from build123d import *

# Parameters (mm, degrees)
SKETCH_1_W               = 114
SKETCH_1_H               = 110
EXTRUDE_2_DEPTH          = 2.5
SKETCH_2_R               = 5
CUT_EXTRUDE_1_DEPTH      = 80.366239674
MIRROR_2_COPY_1_SKETCH_R = 5
MIRROR_2_COPY_1_DEPTH    = 80.366239674
HOLE_WIZARD_M4_1_D       = 3.3
HOLE_WIZARD_M8_3_D       = 6.8
SKETCH_8_R               = 4
CUT_EXTRUDE_2_DEPTH      = 80.366239674
HOLE_WIZARD_M8_4_D       = 6.8


with BuildPart() as part:
    # 草图1 → 凸台-拉伸2 (new, symmetric)
    with BuildSketch(Plane.XY):
        Rectangle(SKETCH_1_W, SKETCH_1_H)
    extrude(amount=EXTRUDE_2_DEPTH, both=True)

    # 草图2 → 切除-拉伸1 (cut, through all)
    with BuildSketch(Plane.XY.offset(2.5)):
        with Locations((-48, 47.5)):
            Circle(SKETCH_2_R)
    cut_extrude_1 = extrude(amount=-CUT_EXTRUDE_1_DEPTH, mode=Mode.SUBTRACT)

    # 镜向1: 切除-拉伸1 across plane
    add(cut_extrude_1.mirror(Plane.ZX), mode=Mode.SUBTRACT)

    # 镜向2: 切除-拉伸1 across plane
    add(cut_extrude_1.mirror(Plane(origin=(0, 0, 0), x_dir=(0, 0, 1), z_dir=(1, 0, 0))), mode=Mode.SUBTRACT)

    # 镜向2 copy 1 sketch → 镜向2 copy 1 (cut, through all)
    with BuildSketch(Plane(origin=(0, 0, 2.5), x_dir=(-1, 0, 0), z_dir=(0, 0, 1))):
        with Locations((-48, 47.5)):
            Circle(MIRROR_2_COPY_1_SKETCH_R)
    extrude(amount=-MIRROR_2_COPY_1_DEPTH, mode=Mode.SUBTRACT)

    # M4 螺纹孔的螺纹孔钻头1 (through all)
    with Locations(Plane(origin=(-23, 9, 2.5), x_dir=(1, 0, 0), z_dir=(0, 0, 1))):
        with Locations((0, 0), (0, -15)):
            hole_wizard_m4_1 = Hole(HOLE_WIZARD_M4_1_D / 2)

    # 镜向4: M4 螺纹孔的螺纹孔钻头1 across plane
    add(hole_wizard_m4_1.mirror(Plane(origin=(0, 0, 0), x_dir=(0, 0, 1), z_dir=(1, 0, 0))), mode=Mode.SUBTRACT)

    # M8 螺纹孔的螺纹孔钻头3 (through all)
    with Locations(Plane(origin=(0, 33, 2.5), x_dir=(1, 0, 0), z_dir=(0, 0, 1))):
        with Locations((0, 0)):
            Hole(HOLE_WIZARD_M8_3_D / 2)

    # 草图8 → 切除-拉伸2 (cut, through all)
    with BuildSketch(Plane.XY.offset(2.5)):
        with Locations((0, 47.5)):
            Circle(SKETCH_8_R)
    extrude(amount=-CUT_EXTRUDE_2_DEPTH, mode=Mode.SUBTRACT)

    # M8 螺纹孔的螺纹孔钻头4 (through all)
    with Locations(Plane(origin=(0, -47.5, 2.5), x_dir=(1, 0, 0), z_dir=(0, 0, 1))):
        with Locations((0, 0)):
            Hole(HOLE_WIZARD_M8_4_D / 2)


solid = part.part
For this review, take the finished solid that the model builds, in its own axes (mm). Coordinates: 2 decimals unless noted, no trailing zeros. Loops run counter-clockwise (first coordinate to the right, second up) from the corner with the lowest first, then second, coordinate; pieces in that order, holes last. Notation, with made-up numbers: (13.25, 23.5) - (18.25, 23.5) arc R13 ccw to (18.25, 43.5) - close; hole circle Ø11 at (40.5, 63). An arc over 180 degrees is marked (long way). Use a Markdown table: item, result. Add a question column.
Item 1: We need section D-D (z = 0.65). Give the number of separate pieces and of enclosed holes in the cut face, and give its area (3 significant figures).
Item 2: Insertion check: pin 1 Ø6 at (x, y) = (0, -47.5) entering from -Z. The pin has a flat end and moves straight along its axis. Give the tip position at first contact, or say it passes through.
Item 3: We need section A-A (x = 0). Give the boundary of the cut face in (y, z), and give its area (3 significant figures).
Item 4: Mouldability with a two-part tool opening along Y and no side actions: class faces 1 (the face through (-1, -55, 0)), 2 (the face through (-57, -1, 0)), 3 (the face through (-21.69, 8, -0.03)), 4 (the face through (-1, 55, 0)) as pulls with the +Y half, pulls with the -Y half, needs draft (parallel to the pull), parting line crosses it, or undercut.
Item 5: We need section B-B (y = -47.5). Give the boundary of the cut face in (x, z), and give its area (3 significant figures).
Item 6: We need section C-C (x = 23). Give the boundary of the cut face in (y, z).
Item 7: For line 1 (Y direction, x = -23, z = 1.4); line 2 (X direction, y = -45.5, z = 2); line 3 (Y direction, x = 1.5, z = 0.2), list the stretches that pass through material, from the lowest coordinate up.
Results list:
| question | item | result |
|---|---|---|
| 1 | separate pieces | 1 |
| 1 | enclosed holes | 11 |
| 1 | area | 12,100 mm^2 |
| 2 | pin 1 | passes through |
| 3 | outline | (-55, -2.5) - (-50.9, -2.5) - (-50.9, 2.5) - (-55, 2.5) - close; (-44.1, -2.5) - (29.6, -2.5) - (29.6, 2.5) - (-44.1, 2.5) - close; (36.4, -2.5) - (43.5, -2.5) - (43.5, 2.5) - (36.4, 2.5) - close; (51.5, -2.5) - (55, -2.5) - (55, 2.5) - (51.5, 2.5) - close |
| 3 | area | 442 mm^2 |
| 4 | face 1 | pulls with the -Y half |
| 4 | face 2 | needs draft |
| 4 | face 3 | undercut |
| 4 | face 4 | pulls with the +Y half |
| 5 | outline | (-57, -2.5) - (-53, -2.5) - (-53, 2.5) - (-57, 2.5) - close; (-43, -2.5) - (-3.4, -2.5) - (-3.4, 2.5) - (-43, 2.5) - close; (3.4, -2.5) - (43, -2.5) - (43, 2.5) - (3.4, 2.5) - close; (53, -2.5) - (57, -2.5) - (57, 2.5) - (53, 2.5) - close |
| 5 | area | 436 mm^2 |
| 6 | outline | (-55, -2.5) - (-7.65, -2.5) - (-7.65, 2.5) - (-55, 2.5) - close; (-4.35, -2.5) - (7.35, -2.5) - (7.35, 2.5) - (-4.35, 2.5) - close; (10.65, -2.5) - (55, -2.5) - (55, 2.5) - (10.65, 2.5) - close |
| 7 | line 1 | y = -55 to -7.65, -4.35 to 7.35, 10.65 to 55 |
| 7 | line 2 | x = -57 to -52.58, -43.42 to -2.75, 2.75 to 43.42, 52.58 to 57 |
| 7 | line 3 | y = -55 to -50.55, -44.45 to 29.95, 36.05 to 43.79, 51.21 to 55 |
